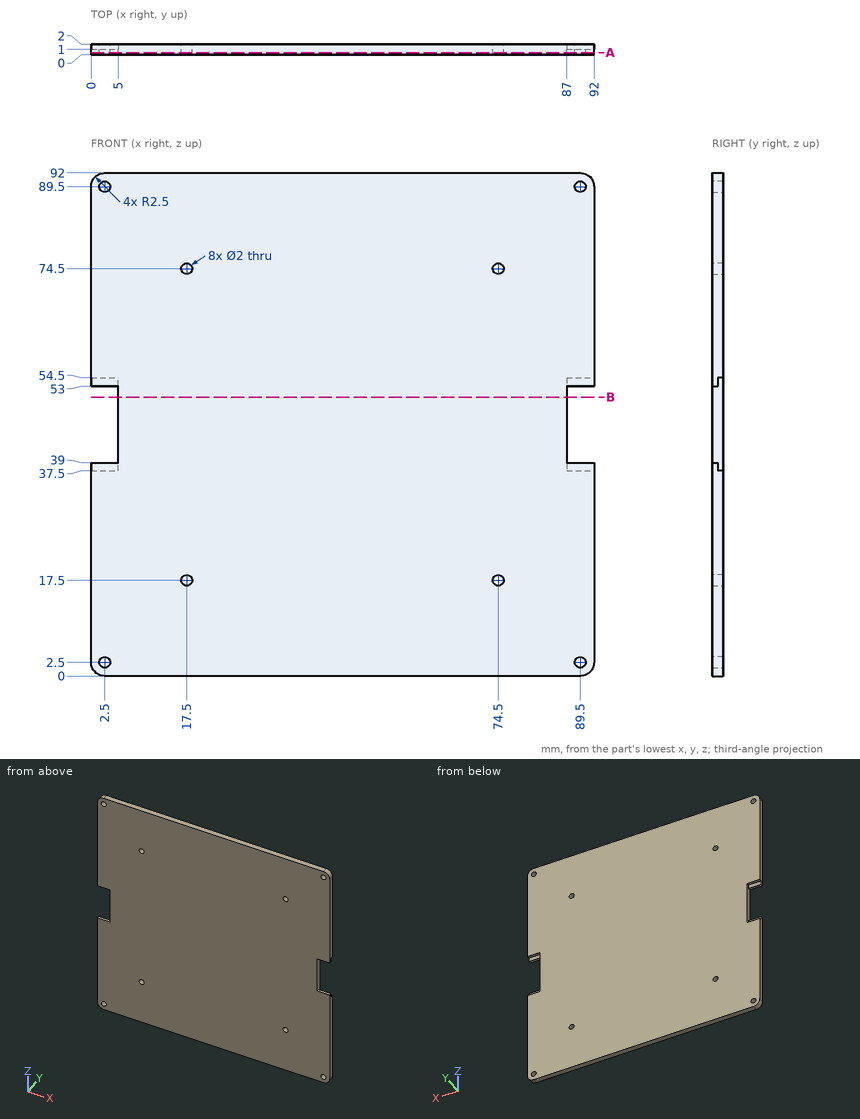
Study the drawing (mm; zero at the part's minimum x, y, z) and answer. Give positions to 0.01 mm unless a question says otherwise; leave off trailing zeros. Write each loop counter-clockwise with the first axis right and the second up, starting at its lowest first coordinate (ties: lowest second). Pieces come first, ordered by that corner, then holes. Notation, with made-up numbers: (63.5, 54) - (115.5, 54) arc R23 cw to (115.5, 72) - close; hole circle Ø9 at (26.5, 32.25). An arc over 180 degrees is marked (long way). Use CSV: the item, a comma, the result in double quotes. Start each with the question number.
(1) Find section B-B (z = 51). Give the vertices of the cut face in (x, y).
(2) Consider line 1 along X through (y, z) = (1.65, 89.5); line 2 along Z through (x, y) = (89.5, 1.25); line 3 along Z through (x, y) = (74.5, 0.5). Determine where each line is inside the solid, lowest interval first.
(3) Given P1, Ø0.8, axis at x = 90, z = 53.5, coming from the +Y side; P2, Ø0.5, axis at x = 1.5, y = 0.5, coming from the -Z side, each flat-ended and moving along its own axis, determine where each tip first touches the part or whether it passes through.
(4) Find section A-A (y = 0.4). Count the separate pieces of the cut face and the enclosed holes in it, plus the area to 3 significant figures.
Findings below:
1,outline,"(5, 0) - (87, 0) - (87, 2) - (5, 2) - close"
2,line 1,"0 to 1.5, 3.5 to 88.5, 90.5 to 92"
2,line 2,"0 to 1.5, 3.5 to 37.5, 54.5 to 88.5, 90.5 to 92"
2,line 3,"0 to 16.5, 18.5 to 73.5, 75.5 to 92"
3,P1,"y = 1"
3,P2,"z = 0.12"
4,separate pieces,"1"
4,enclosed holes,"8"
4,area,"8,290 mm2"
